Study the drawing (mm; zero at the part's minimum x, y, z) and answer. A direction names the side the tool comes from. Give positions to 0.01 mm unless a question says otherwise; leave off trailing zeros. Write each loop counter-clockwise with the first axis right and the second up, starting at its lowest first coordinate (ties: lowest second). Pieces come first, ordered by that corner, then holes.
1) Given pin 1 Ø6 at (x, y) = (54.5, 3.5) entering from +Z (1 decimal); pin 2 Ø1 at (x, z) = (31.5, 17.5) entering from -Y; pin 3 Ø3 at (y, z) = (2, 4.5) entering from +X; pin 4 Ø4 at (y, z) = (7, 27) entering from +X, each flat-ended and moving along its own axis, determine where each tip first touches the part or whether it passes through.
2) Find section C-C (y = 2.75). Determine the outline of the cut face in (x, z) (1 decimal), plus the area to 3 significant figures.
3) Find section B-B (z = 28.5). Determine the outline of the cut face in (x, y), plus the area to 3 significant figures.
4) Find section A-A (x = 35). Determine the outline of the cut face in (y, z).
5) Find section D-D (z = 19). Determine the outline of the cut face in (x, y).
6) A tool of negligible diameter and unlimited length cuts with its end or side. For the marked faces 5, 6 and 7, from which of +Z, -Z, +X, -X, +Y, -Y can it reach the whole face along a straight path? Write none if from no direction.
7) Straight lines are drawn through the part: probe 1 along X at (y, z) = (5.5, 7.5); probe 2 along X at (y, z) = (2.25, 29) (1 decimal); probe 3 along Z at (x, y) = (3.5, 8.75). For each, find the intervals that lie inside material, in ascending order.
8) Determine the mould class of the marked faces 1, 2, 3 and 4 for opening direction Z: pulls with the +Z half, pulls with the -Z half, needs draft (parallel to the pull), parting line crosses it, or undercut.
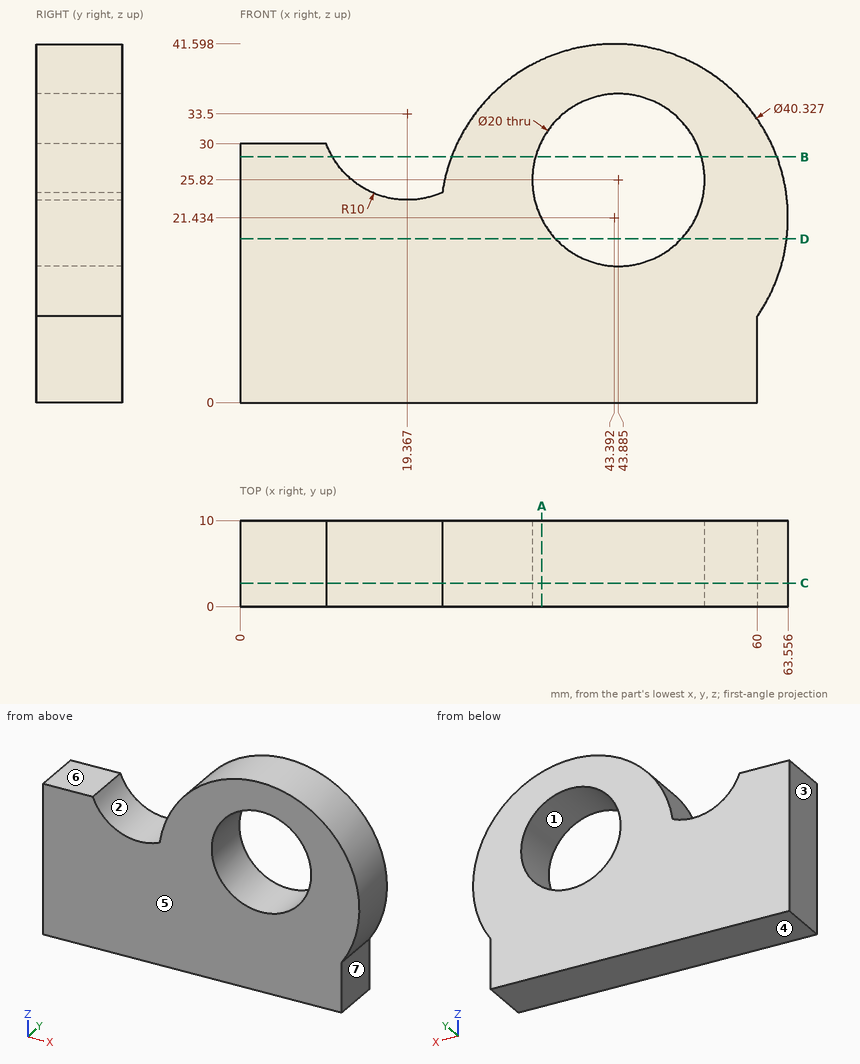
Results:
1. pin 1: stops at z = 39.9
1. pin 2: stops at y = 0
1. pin 3: stops at x = 60
1. pin 4: stops at x = 63.24
2. outline: (0, 0) - (60, 0) - (60, 10) arc R20.2 ccw (long way) to (23.4, 24.4) arc R10 cw to (10, 30) - (0, 30) - close; hole circle Ø20 at (43.9, 25.8)
2. area: 1,770 mm2
3. outline: (0, 0) - (10.71, 0) - (10.71, 10) - (0, 10) - close; (24.51, 0) - (34.25, 0) - (34.25, 10) - (24.51, 10) - close; (53.52, 0) - (62.28, 0) - (62.28, 10) - (53.52, 10) - close
3. area: 292 mm2
4. outline: (0, 0) - (10, 0) - (10, 21.23) - (0, 21.23) - close; (0, 30.41) - (10, 30.41) - (10, 39.77) - (0, 39.77) - close
5. outline: (0, 0) - (36.57, 0) - (36.57, 10) - (0, 10) - close; (51.2, 0) - (63.41, 0) - (63.41, 10) - (51.2, 10) - close
6. face 5: +Z, -Z, +X, -X, -Y
6. face 6: +Z, -X, +Y, -Y
6. face 7: -Z, +X, +Y, -Y
7. probe 1: x = 0 to 60
7. probe 2: x = 0 to 10.4, 24.7 to 34.4, 53.4 to 62.1
7. probe 3: z = 0 to 30
8. face 1: undercut
8. face 2: pulls with the +Z half
8. face 3: needs draft
8. face 4: pulls with the -Z half
